Part model, mm, in its own coordinate system. A direction names the side the tool comes from. Round coordinates to 2 decimals unless told otherwise and drop trailing zeros. Loops run counter-clockwise (first coordinate to the right, second up) from the corner with the lowest first, then second, coordinate; pieces in that order, holes last.
1) Band-saw the part on C-C, the plane x = 118. Write the cut outline in (y, z), then the cut area to 3 significant figures.
2) Probe line 1 (Y direction, x = -0.5, z = 445); line 2 (X direction, y = 201.5, z = 417.5); line 3 (Z direction, x = 936, y = 506). List the from-to ranges inside material, lowest first.
3) 3-axis set-ups, long thin cutter, end or side, ignore diameter. For faces 1 (the flat face through (684, -71.674, 301)), 2 (the flat face through (-66.924, 379, 313)): which of +Z, -Z, +X, -X, +Y, -Y reach the whole face in a straight line?
4) Mould opens along Y. For faces 3 (the flat face through (684, 842.726, 301)), 4 (the flat face through (684, 842.345, 313)), 5 (the flat face through (684, 392, 0)), 6 (the flat face through (684, -71.293, 313)) say: +Y half, -Y half, draft (parallel to the pull), parting line (faces both ways), or undercut.
5) Band-saw the part on B-B, the plane y = 235. Write the cut outline in (x, z), then the cut area to 3 significant figures.
6) Band-saw the part on A-A, the plane z = 121. Write the cut outline in (x, y), then the cut area to 3 significant figures.
7) Drop a flat-ended pin along its axis: P1, Ø6, axis at x = 1177, y = 28.5, coming from the +Z side. Give the stop position or say it passes through.
from build123d import *

# Parameters (mm, degrees)
F1_W     = 1524
F1_H     = 914.4
F1_W_2   = 1522.73
F1_H_2   = 913.638
F2_DEPTH = 609.6
F0_W     = 1524
F0_H     = 914.4
F3_DEPTH = 25.4
F6_DEPTH = 63.5


with BuildPart() as f2:
    # F1 (on face) → F2 (new body)
    with BuildSketch(Plane.XY):
        with Locations((694.4408099055, 385.5257871866)):
            Rectangle(F1_W, F1_H)
        with Locations((694.4408099055, 385.5257871866)):
            Rectangle(F1_W_2, F1_H_2, mode=Mode.SUBTRACT)
    extrude(amount=F2_DEPTH)

    # F1 (on face) + F0 (on Top) → F3 (join)
    with BuildSketch(Plane.XY):
        with Locations((694.4408099055, 385.5257871866)):
            Rectangle(F1_W_2, F1_H_2)
    with BuildSketch(Plane.XY):
        with Locations((694.4408099055, 385.5257871866)):
            Rectangle(F0_W, F0_H)
    extrude(amount=F3_DEPTH)

    # F5 (on mid) → F6 (join, symmetric)
    with BuildSketch(Plane(origin=(-0.3153710141, -0.1892226085, 302.7561735554), x_dir=(0.9999994575, -6.51e-07, 0.0010416657), z_dir=(0.0010416659, 0.0006249995, -0.9999992622))):
        with BuildLine():
            ThreePointArc((1482.474916731, -157.6878010367), (1475.0354348197, -139.727294641), (1457.0749332675, -132.2878010367))
            Line((1457.0749332675, -132.2878010367), (1457.074916731, -157.6878010367))
            Line((1457.074916731, -157.6878010367), (1457.0749001946, -183.0878010367))
            ThreePointArc((1457.0749001946, -183.0878010367), (1475.0354231266, -175.6483191253), (1482.474916731, -157.6878010367))
        make_face()
        with BuildLine():
            ThreePointArc((1482.4747680271, -386.097211777), (1475.0352861157, -368.1367053814), (1457.0747845635, -360.697211777))
            Line((1457.0747845635, -360.697211777), (1457.0747680271, -386.097211777))
            Line((1457.0747680271, -386.097211777), (1457.0747514906, -411.497211777))
            ThreePointArc((1457.0747514906, -411.497211777), (1475.0352744227, -404.0577298657), (1482.4747680271, -386.097211777))
        make_face()
        with BuildLine():
            ThreePointArc((1482.4746193231, -614.5066225174), (1475.0351374118, -596.5461161218), (1457.0746358596, -589.1066225174))
            Line((1457.0746358596, -589.1066225174), (1457.0746193231, -614.5066225174))
            Line((1457.0746193231, -614.5066225174), (1457.0746027867, -639.9066225174))
            ThreePointArc((1457.0746027867, -639.9066225174), (1475.0351257188, -632.467140606), (1482.4746193231, -614.5066225174))
        make_face()
        with BuildLine():
            Line((1457.0746193231, -614.5066225174), (1457.0746358596, -589.1066225174))
            ThreePointArc((1457.0746358596, -589.1066225174), (1431.6746193231, -614.5066059809), (1457.0746027867, -639.9066225174))
            Line((1457.0746027867, -639.9066225174), (1457.0746193231, -614.5066225174))
        make_face()
        with BuildLine():
            Line((1457.0747680271, -386.097211777), (1457.0747845635, -360.697211777))
            ThreePointArc((1457.0747845635, -360.697211777), (1431.6747680271, -386.0971952406), (1457.0747514906, -411.497211777))
            Line((1457.0747514906, -411.497211777), (1457.0747680271, -386.097211777))
        make_face()
        with BuildLine():
            Line((1457.074916731, -157.6878010367), (1457.0749332675, -132.2878010367))
            ThreePointArc((1457.0749332675, -132.2878010367), (1431.674916731, -157.6877845002), (1457.0749001946, -183.0878010367))
            Line((1457.0749001946, -183.0878010367), (1457.074916731, -157.6878010367))
        make_face()
    extrude(amount=F6_DEPTH, both=True)


solid = f2.part
Reported:
1. outline: (-71.67, 0) - (842.73, 0) - (842.73, 609.6) - (842.34, 609.6) - (842.34, 25.4) - (-71.29, 25.4) - (-71.29, 609.6) - (-71.67, 609.6) - close
1. area: 23,700 mm2
2. line 1: y = -71.67 to -71.29, 842.34 to 842.73
2. line 2: x = -67.56 to -66.92, 1455.81 to 1456.44
2. line 3: z = 0 to 25.4
3. face 1: +Z, -Z, +X, -X, -Y
3. face 2: +Z
4. face 3: +Y half
4. face 4: undercut
4. face 5: draft
4. face 6: undercut
5. outline: (-67.56, 0) - (1456.44, 0) - (1456.44, 609.6) - (1455.81, 609.6) - (1455.81, 25.4) - (-66.92, 25.4) - (-66.92, 609.6) - (-67.56, 609.6) - close
5. area: 39,500 mm2
6. outline: (-67.56, -71.67) - (1456.44, -71.67) - (1456.44, 842.73) - (-67.56, 842.73) - close; hole (-66.92, -71.29) - (1455.81, -71.29) - (1455.81, 842.34) - (-66.92, 842.34) - close
6. area: 2,320 mm2
7. P1: stops at z = 25.4
